Verification items for this drawing (mm, ordinates from the low corner). Give positions to 0.01 mm unless a question says otherwise; leave off trailing zeros. Loops run counter-clockwise (first coordinate to the right, second up) from the corner with the lowest first, then second, coordinate; pieces in that order, holes last. Notation, with made-up numbers: (81.5, -4) -> (115.5, -4) arc R20 cw to (115.5, 8) -> close; hole circle Ø4 at (22, 53). An arc over 180 degrees is marked (long way). Use one line per item in the form item = value. Start each with the question number.
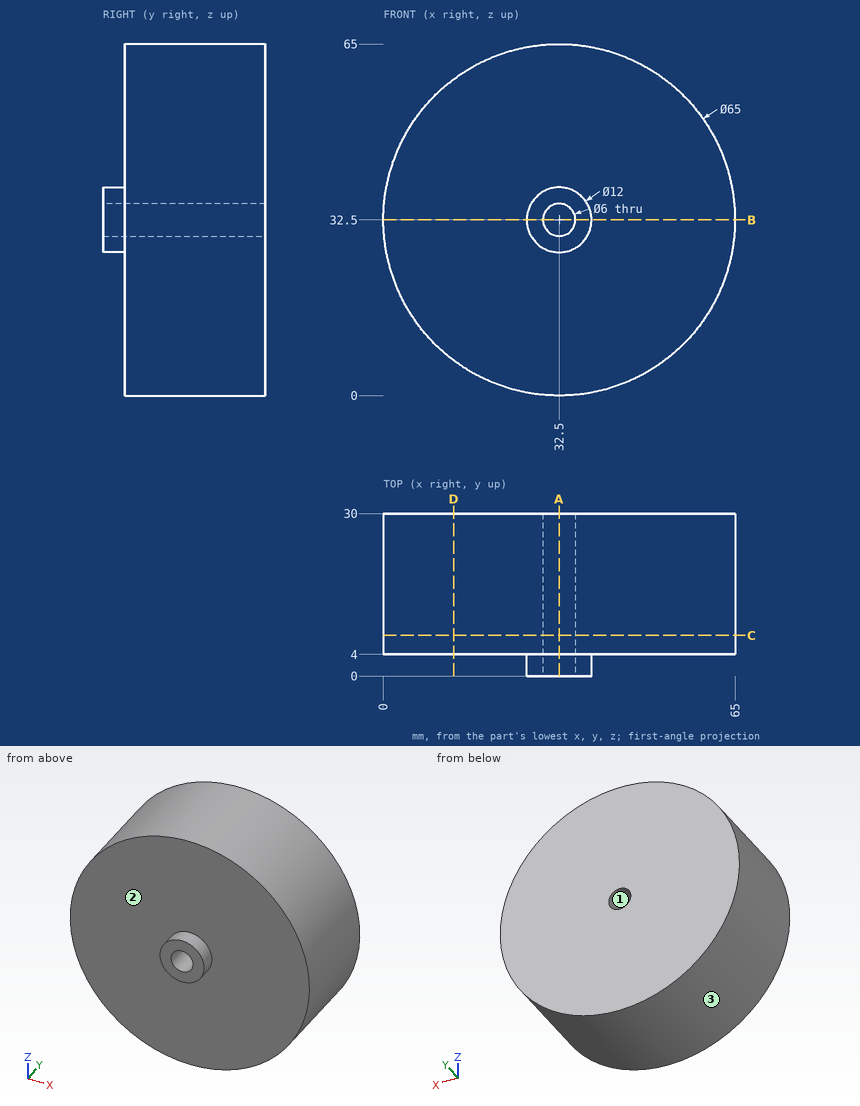
Item 1: Sectioned sample at A-A, the plane x = 32.5. Enter the section's corners in (y, z).
Item 2: Material ranges on line 1 (X direction, y = 23.5, z = 32.5); line 2 (Y direction, x = 19.5, z = 50); line 3 (Z direction, x = 13, y = 20), recorded low to high.
Item 3: Sectioned sample at D-D, the plane x = 13. Enter the section's corners in (y, z), and give its area (3 significant figures).
Item 4: Sectioned sample at C-C, the plane y = 7.5. Enter the section's corners in (x, z), and give its area (3 significant figures).
Item 5: Draft check along Z on the marked faces 1, 2 and 3. Enter one of: +Z half, -Z half, draft (parallel to the pull), parting line (faces both ways), or undercut.
Item 6: Sectioned sample at B-B, the plane z = 32.5. Enter the section's corners in (x, y), and give its area (3 significant figures).
Item 7: Gauge pin test, flat ends, axial feed: pin 1 Ø10 at (x, z) = (54.5, 36) entering from -Y; pin 2 Ø2 at (x, y) = (12, 19.5) entering from -Z; pin 3 Ø6 at (y, z) = (4, 11) entering from -X; pin 4 Ø5.5 at (x, z) = (32.5, 32.5) entering from +Y. Record the tip position at first contact, or that the pin passes through.
Outcome:
q1.outline = (0, 26.5) -> (4, 26.5) -> (4, 0) -> (30, 0) -> (30, 29.5) -> (0, 29.5) -> close; (0, 35.5) -> (30, 35.5) -> (30, 65) -> (4, 65) -> (4, 38.5) -> (0, 38.5) -> close
q2.line_1 = 0 to 29.5, 35.5 to 65
q2.line_2 = 4 to 30
q2.line_3 = 6.5 to 58.5
q3.outline = (4, 6.5) -> (30, 6.5) -> (30, 58.5) -> (4, 58.5) -> close
q3.area = 1,350 mm^2
q4.outline = circle Ø65 at (32.5, 32.5); hole circle Ø6 at (32.5, 32.5)
q4.area = 3,290 mm^2
q5.face_1 = undercut
q5.face_2 = draft
q5.face_3 = parting line
q6.outline = (0, 4) -> (26.5, 4) -> (26.5, 0) -> (29.5, 0) -> (29.5, 30) -> (0, 30) -> close; (35.5, 0) -> (38.5, 0) -> (38.5, 4) -> (65, 4) -> (65, 30) -> (35.5, 30) -> close
q6.area = 1,560 mm^2
q7.pin_1 = 4
q7.pin_2 = 6.5
q7.pin_3 = 5.78
q7.pin_4 = through
